Input: part model. Units: mm. Frame: model coordinates. A direction names the side the tool comes from. Round coordinates to 2 decimals unless told otherwise and drop trailing zeros. Order: outer loops, then holes, each group sorted by start corner. A loop starts at its lowest first (then second) coordinate and runs counter-clockwise, first axis right, second up. Notation, with made-up numbers: (7, 0) - (65, 0) arc R17 cw to (65, 14) - close; hole circle Ø3 at (78, 45.25). An arc over 180 degrees is marked (long way). One line per item, written item: value. Start each with the question number.
from build123d import *

# Parameters (mm, degrees)
SKETCH1_W               = 76.2
SKETCH1_H               = 50.8
BOSS_EXTRUDE1_DEPTH     = 9.525
F_1_4_CLEARANCE_HOLE1_D = 6.7564
CUT_EXTRUDE1_DEPTH      = 65.210401221
SKETCH5_R               = 1.190625
CUT_EXTRUDE2_DEPTH      = 47.770670564
F_8_CLEARANCE_HOLE1_D   = 4.4958
SKETCH8_R               = 5.08
CUT_EXTRUDE3_DEPTH      = 4.7625
SKETCH9_R               = 3.81
CUT_EXTRUDE4_DEPTH      = 4.7625


with BuildPart() as part:
    # Sketch1 → Boss-Extrude1 (new body)
    with BuildSketch(Plane(origin=(0, 0, 0), x_dir=(1, 0, 0), z_dir=(0, 1, 0))):
        Rectangle(SKETCH1_W, SKETCH1_H)
    extrude(amount=BOSS_EXTRUDE1_DEPTH)

    # 1/4 Clearance Hole1 (through all)
    with Locations(Plane(origin=(0, 9.525, 0), x_dir=(1, 0, 0), z_dir=(0, 1, 0))):
        with Locations((0, 14.61008), (-13.86078, -10.78992), (13.86078, -10.78992)):
            Hole(F_1_4_CLEARANCE_HOLE1_D / 2)

    # Sketch4 → Cut-Extrude1 (cut, through all)
    with BuildSketch(Plane.XY.offset(25.4)):
        with BuildLine():
            Line((-27.6225, 9.525), (-18.0975, 9.525))
            ThreePointArc((-18.0975, 9.525), (-22.86, 4.7625), (-27.6225, 9.525))
        make_face()
        with BuildLine():
            Line((18.0975, 9.525), (27.6225, 9.525))
            ThreePointArc((27.6225, 9.525), (22.86, 4.7625), (18.0975, 9.525))
        make_face()
    extrude(amount=-CUT_EXTRUDE1_DEPTH, mode=Mode.SUBTRACT)

    # Sketch5 → Cut-Extrude2 (cut, through all)
    with BuildSketch(Plane(origin=(0, 9.525, 0), x_dir=(1, 0, 0), z_dir=(0, 1, 0))):
        with Locations(Location((0, -3.175, 0), (0, 0, 270))):
            Circle(SKETCH5_R)
    extrude(amount=-CUT_EXTRUDE2_DEPTH, mode=Mode.SUBTRACT)

    # #8 Clearance Hole1 (through all)
    with Locations(Plane(origin=(0, 9.525, 0), x_dir=(1, 0, 0), z_dir=(0, 1, 0))):
        with Locations((-33.02, 15.875), (-33.02, -15.875), (33.02, -15.875), (33.02, 15.875), (-12.7, 15.875), (12.7, 15.875), (0, -15.875)):
            Hole(F_8_CLEARANCE_HOLE1_D / 2)

    # Sketch8 → Cut-Extrude3 (cut)
    with BuildSketch(Plane.XZ):
        with Locations(Location((-13.86078, 10.78992, 0), (0, 0, 270))):
            Circle(SKETCH8_R)
        with Locations(Location((13.86078, 10.78992, 0), (0, 0, 270))):
            Circle(SKETCH8_R)
        with Locations(Location((0, -14.61008, 0), (0, 0, 270))):
            Circle(SKETCH8_R)
    extrude(amount=-CUT_EXTRUDE3_DEPTH, mode=Mode.SUBTRACT)

    # Sketch9 → Cut-Extrude4 (cut)
    with BuildSketch(Plane.XZ):
        with Locations(Location((-33.02, 15.875, 0), (0, 0, 270))):
            Circle(SKETCH9_R)
        with Locations(Location((0, 15.875, 0), (0, 0, 270))):
            Circle(SKETCH9_R)
        with Locations(Location((33.02, 15.875, 0), (0, 0, 270))):
            Circle(SKETCH9_R)
        with Locations(Location((33.02, -15.875, 0), (0, 0, 270))):
            Circle(SKETCH9_R)
        with Locations(Location((12.7, -15.875, 0), (0, 0, 270))):
            Circle(SKETCH9_R)
        with Locations(Location((-12.7, -15.875, 0), (0, 0, 270))):
            Circle(SKETCH9_R)
        with Locations(Location((-33.02, -15.875, 0), (0, 0, 270))):
            Circle(SKETCH9_R)
    extrude(amount=-CUT_EXTRUDE4_DEPTH, mode=Mode.SUBTRACT)


solid = part.part
Item 1: First-contact query: pin 1 Ø7 at (x, z) = (0, 15.875) entering from -Y; pin 2 Ø1 at (x, y) = (-19, 8) entering from +Z. Flat tips, straight axial feed; report the tip coordinate or a pass-through.
Item 2: Section query A-A on x = -33.02. Return loops of the section in (y, z) (1 decimal).
Item 3: Reachability of faces 4 (the face through (-35, 4.762, -18)), 5 (the face through (-1, 0, 0)) from +Z, -Z, +X, -X, +Y, -Y: full face, straight path, thin tool, end or side. Return the list, or none.
Item 4: Section query B-B on y = 2.25. Give the number of separate pieces and of enclosed holes in the cut face, and give its area (3 significant figures).
Item 5: Pull-direction query (X, two-part tool) for faces 1 (the face through (10.5, 4.762, 9.7)), 2 (the face through (33, 9.525, 0)), 3 (the face through (0.052, 4.829, 1.986)); classes: released by +X, released by -X, zero draft, split by the parting line, or undercut.
Item 6: Section query C-C on z = -5. Return loops of the section in (x, y) (1 decimal).
Item 7: Line query: L1, parallel to Z at x = -33.02, y = 6; L2, parallel to X at y = 8, z = -20.5; L3, parallel to X at y = 3.5, z = 12.5. Output: solid intervals per line, ascending.
Geometry results:
1. pin 1: stops at y = 4.76
1. pin 2: passes through
2. outline: (0, -25.4) - (9.5, -25.4) - (9.5, -18.1) - (4.8, -18.1) - (4.8, -19.7) - (0, -19.7) - close; (0, -12.1) - (4.8, -12.1) - (4.8, -13.6) - (9.5, -13.6) - (9.5, 13.6) - (4.8, 13.6) - (4.8, 12.1) - (0, 12.1) - close; (0, 19.7) - (4.8, 19.7) - (4.8, 18.1) - (9.5, 18.1) - (9.5, 25.4) - (0, 25.4) - close
3. face 4: -Y
3. face 5: +Z, -Z, +X, -X, -Y
4. separate pieces: 1
4. enclosed holes: 11
4. area: 3,300 mm^2
5. face 1: undercut
5. face 2: zero draft
5. face 3: undercut
6. outline: (-38.1, 0) - (38.1, 0) - (38.1, 9.5) - (27.6, 9.5) arc R4.8 cw to (18.1, 9.5) - (-18.1, 9.5) arc R4.8 cw to (-27.6, 9.5) - (-38.1, 9.5) - close
7. L1: z = -25.4 to -18.12, -13.63 to 13.63, 18.12 to 25.4
7. L2: x = -38.1 to -27.37, -18.35 to 18.35, 27.37 to 38.1
7. L3: x = -38.1 to -34.79, -31.25 to -18.64, -9.08 to -1.77, 1.77 to 9.08, 18.64 to 31.25, 34.79 to 38.1
